Can you work these out from the model? Positions are in its coordinate system, mm. Face numbers are marked on the shaded views. Round coordinates to 2 decimals unless told otherwise and drop trailing zeros. Order: outer loops, then holes, each group sorted by start corner. A loop starts at its lowest first (then second) coordinate and runs counter-clockwise, first axis right, second up.
Q1. If I drill on line 1 (X direction, y = 1.15, z = -1.4); line 2 (Z direction, x = -6, y = 0.05); line 3 (Y direction, x = -10.75, z = -1.3), over which ranges is the centre line in solid material (lowest first)?
Q2. If we section it at A-A (x = -1.75): Please give me the cut outline in (y, z), plus the area to 3 significant figures.
Q3. Will these pins go through, and if not, where does the flat tip stop? P1, Ø1, axis at y = -1, z = -0.5, coming from the -X side; P2, Ø3, axis at x = -3, y = -0.5, coming from the -Z side.
Q4. We'd pull the mould along Z, two halves only. Please class the marked faces 1, 2 and 3: pulls with the +Z half, pulls with the -Z half, needs draft (parallel to the pull), parting line crosses it, or undercut.
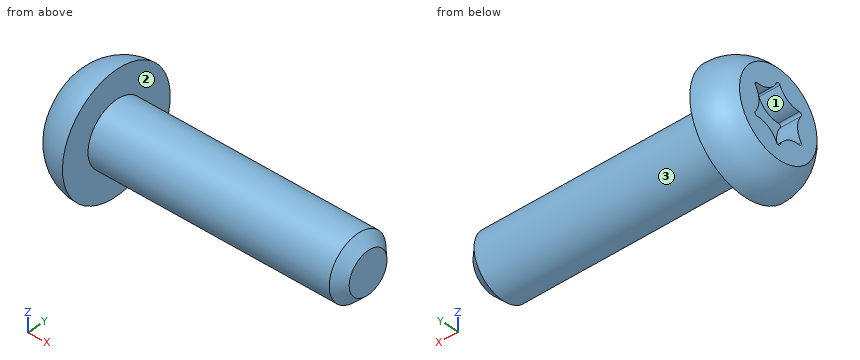
from build123d import *

# Parameters (mm, degrees)
CHAMFER1_SIZE      = 0.5
CUT_EXTRUDE1_DEPTH = 1


with BuildPart() as part:
    # Sketch2 → Revolve1 (revolve)
    with BuildSketch(Plane(origin=(0, 0, 0), x_dir=(1, 0, 0), z_dir=(0, 1, 0)), mode=Mode.PRIVATE) as revolve1_sk:
        with BuildLine():
            Line((0, 0), (0, 1.5))
            Line((0, 1.5), (-12, 1.5))
            Line((-12, 1.5), (-12, 2.85))
            ThreePointArc((-12, 2.85), (-12.917065968, 2.639177072), (-13.65, 2.049038106))
            Line((-13.65, 2.049038106), (-13.65, 0))
            Line((-13.65, 0), (0, 0))
        make_face()
    revolve(revolve1_sk.sketch.rotate(Axis((-13.65, 0, 0), (1, 0, 0)), 180), axis=Axis((-13.65, 0, 0), (1, 0, 0)))

    # Chamfer1
    chamfer1_edges = [part.edges().sort_by_distance(p)[0] for p in [
        (0, 0, -1.5),
    ]]
    chamfer(chamfer1_edges, length=CHAMFER1_SIZE)

    # Sketch4 → Cut-Extrude1 (cut)
    with BuildSketch(Plane.ZY.offset(13.65)):
        with BuildLine():
            ThreePointArc((-1.342027284, 0.090739778), (-0.883315009, 0.509982158), (-0.749596595, 1.116859832))
            ThreePointArc((-0.749596595, 1.116859832), (-0.7, 1.212435565), (-0.592430689, 1.20759961))
            ThreePointArc((-0.592430689, 1.20759961), (0, 1.019964317), (0.592430689, 1.20759961))
            ThreePointArc((0.592430689, 1.20759961), (0.7, 1.212435565), (0.749596595, 1.116859832))
            ThreePointArc((0.749596595, 1.116859832), (0.883315009, 0.509982158), (1.342027284, 0.090739778))
            ThreePointArc((1.342027284, 0.090739778), (1.4, 0), (1.342027284, -0.090739778))
            ThreePointArc((1.342027284, -0.090739778), (0.883315009, -0.509982158), (0.749596595, -1.116859832))
            ThreePointArc((0.749596595, -1.116859832), (0.7, -1.212435565), (0.592430689, -1.20759961))
            ThreePointArc((0.592430689, -1.20759961), (0, -1.019964317), (-0.592430689, -1.20759961))
            ThreePointArc((-0.592430689, -1.20759961), (-0.7, -1.212435565), (-0.749596595, -1.116859832))
            ThreePointArc((-0.749596595, -1.116859832), (-0.883315009, -0.509982158), (-1.342027284, -0.090739778))
            ThreePointArc((-1.342027284, -0.090739778), (-1.4, 0), (-1.342027284, 0.090739778))
        make_face()
    extrude(amount=-CUT_EXTRUDE1_DEPTH, mode=Mode.SUBTRACT)


solid = part.part
Solution:
1. line 1: x = -13.65 to -12
1. line 2: z = -1.5 to 1.5
1. line 3: y = -0.75 to 0.75
2. outline: circle Ø3 at (0, 0)
2. area: 7.07 mm2
3. P1: stops at x = -13.65
3. P2: stops at z = -1.5
4. face 1: undercut
4. face 2: needs draft
4. face 3: parting line crosses it
